Autodesk Inventor part; units mm, degrees
ref_plane "YZ Plane" through (0, 0, 0) normal (1, 0, 0) x (0, 1, 0)
ref_plane "XZ Plane" through (0, 0, 0) normal (0, 1, 0) x (-1, 0, 0)
ref_plane "XY Plane" through (0, 0, 0) normal (0, 0, 1) x (1, 0, 0)
sketch "Sketch1" plane through (0, 0, 0) normal (0, 0, 1) x (1, 0, 0)
  line L0 (0, 0) -> (9.525, 0)
  line L1 (9.525, 0) -> (9.525, 60.325)
  line L2 (9.525, 60.325) -> (0, 60.325)
  line L3 (0, 60.325) -> (0, 0)
  circle A0 centre (4.7625, 55.5625) radius 4.7625
  circle A1 centre (4.7625, 4.7625) radius 4.7625
  point P0 (4.7625, 0)
  dimension "d0" = 50.8
  dimension "d3" = 9.525
extrude "Extrusion1" add sketch "Sketch1" along normal blind 3.175
hole "Hole1" at (4.7625, 4.7625, 0) at (4.7625, 55.5625, 0) direction (0, 0, 1) diameter 3 end through all
fillet "Fillet1" radius 4.7625 4 edges at (9.525, 0, 1.5875) (0, 0, 1.5875) (0, 60.325, 1.5875) (9.525, 60.325, 1.5875)
sketch "Sketch2" plane through (0, 0, 3.175) normal (0, 0, 1) x (1, 0, 0)
  circle A0 centre (4.7625, 4.7625) radius 1.5
  circle A1 centre (4.7625, 55.5625) radius 1.5
  arc A2 (9.525, 55.5625) -> (0, 55.5625) centre (4.7625, 55.5625) ccw
  line L0 (0, 55.5625) -> (0, 4.7625)
  arc A3 (0, 4.7625) -> (9.525, 4.7625) centre (4.7625, 4.7625) ccw
  line L1 (9.525, 4.7625) -> (9.525, 55.5625)
  point P0 (0, 0)
equation "\"d13\" = 0.5 * d3"
properties part number "Linkage"
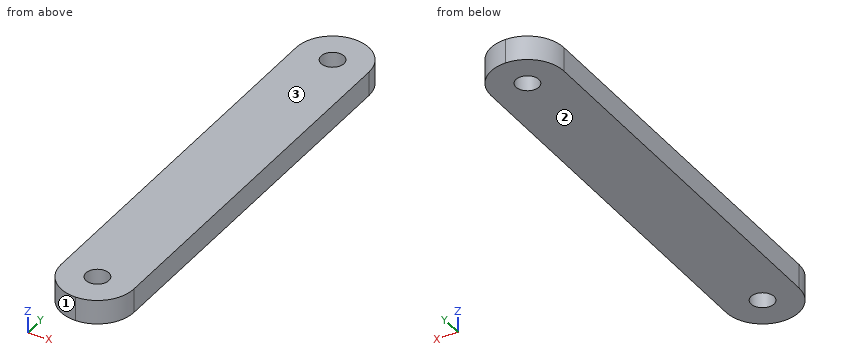
CAD build for the part. Positions are in the model's coordinates, mm. Face numbers are marked on the shaded views. Coordinates: 2 decimals unless noted, no trailing zeros. Write each loop counter-clockwise with the first axis right and the second up, starting at its lowest first coordinate (ties: lowest second). Pieces come first, ordered by that corner, then holes. Notation, with made-up numbers: (-35.75, -9.5) -> (-17.75, -9.5) arc R24 ccw to (-17.75, 11.5) -> close; hole circle Ø9 at (-23.5, 12). An arc over 180 degrees is marked (long way). Use CSV: the item, a comma, the result in double quotes. Start each with the question number.
Item 1: Band-saw the part on B-B, the plane z = 0.95. Give the number of separate pieces and of enclosed holes in the cut face, plus the area to 3 significant figures.
Item 2: Band-saw the part on A-A, the plane x = 4.25. Write the cut outline in (y, z) (3 decimals), plus the area to 3 significant figures.
Item 3: Wall check: probe 1 along Y at (x, z) = (4.75, 1.3); probe 2 along Y at (x, z) = (5, 2); probe 3 along Y at (x, z) = (7.25, 0.55). Give the ranges that are in metal, low to high.
Item 4: Drop a flat-ended pin along its axis: P1, Ø5, axis at x = 4.76, y = 55.56, coming from the -Z side. Give the stop position or say it passes through.
Item 5: Band-saw the part on D-D, the plane x = 8. Write the cut outline in (y, z) (3 decimals).
Item 6: Two-plate mould, pull along Z, no slides. Class the marked faces 1, 2 and 3: +Z half, -Z half, draft (parallel to the pull), parting line (faces both ways), or undercut.
Item 7: Band-saw the part on C-C, the plane x = 1.5. Write the cut outline in (y, z) (3 decimals), plus the area to 3 significant figures.
Response values:
1,separate pieces,"1"
1,enclosed holes,"2"
1,area,"541 mm2"
2,outline,"(0.028, 0) -> (3.353, 0) -> (3.353, 3.175) -> (0.028, 3.175) -> close; (6.172, 0) -> (54.153, 0) -> (54.153, 3.175) -> (6.172, 3.175) -> close; (56.972, 0) -> (60.297, 0) -> (60.297, 3.175) -> (56.972, 3.175) -> close"
2,area,"173 mm2"
3,probe 1,"y = 0 to 3.26, 6.26 to 54.06, 57.06 to 60.32"
3,probe 2,"y = 0.01 to 3.28, 6.24 to 54.08, 57.04 to 60.32"
3,probe 3,"y = 0.7 to 59.62"
4,P1,"stops at z = 0"
5,outline,"(1.269, 0) -> (59.056, 0) -> (59.056, 3.175) -> (1.269, 3.175) -> close"
6,face 1,"draft"
6,face 2,"-Z half"
6,face 3,"+Z half"
7,outline,"(1.293, 0) -> (59.032, 0) -> (59.032, 3.175) -> (1.293, 3.175) -> close"
7,area,"183 mm2"
